Check sheet for the modelled part. Datum: model origin and axes. Units: mm. A direction names the side the tool comes from. Round coordinates to 2 decimals unless told otherwise and drop trailing zeros. Order: outer loops, then holes, each group sorted by start corner. A loop starts at its lowest first (then second) coordinate and runs counter-clockwise, first axis right, second up.
(1) Depth check by flat-ended pin: pin 1 (5 mm diameter, centred on x = -10.5, z = 37.5, fed in from -Y); pin 2 (12 mm diameter, centred on x = -43.5, z = 7.5, fed in from +Y). Enter the tip coordinate at first touch or a pass-through.
(2) Thickness scan on probe 1 along Z at (x, y) = (-9, 74); probe 2 along Z at (x, y) = (-75, 3); probe 3 along Y at (x, z) = (-89.5, 12.5). Record the ranges inside material, lowest first.
(3) Sectioned sample at D-D, the plane z = 8. Enter the section's corners in (x, y).
(4) Mould release check, pull along X, two halves, no side actions. Record for faces 1 (the flat face through (-17, 35, 60)), 2 (the flat face through (-15, 15, 30)), 3 (the flat face through (0, 44, 9)): released by +X, released by -X, zero draft, split by the parting line, or undercut.
(5) Sectioned sample at A-A, the plane x = -75. Enter the section's corners in (y, z).
(6) Tool access check on faces 4 (the flat face through (-20, 51, 30)), 5 (the flat face through (-12, 90, 30)), 6 (the cylindrical face through (-17.496, 20.07, 30.385)). Record the directions out of +Z, -Z, +X, -X, +Y, -Y that give a thin tool (end or side, any length) a straight path to the whole face; none if there is none.
(7) Sectioned sample at B-B, the plane z = 40. Enter the section's corners in (x, y), and give its area (3 significant figures).
(8) Sectioned sample at C-C, the plane y = 37. Enter the section's corners in (x, z), and give its area (3 significant figures).
```python
from build123d import *

# Parameters (mm, degrees)
F1_DEPTH = 60
F3_DEPTH = 90.001
F4_R     = 3.75
F5_DEPTH = 10.001
F6_W     = 10
F6_H     = 3


with BuildPart() as f1:
    # F0 (on Top) → F1 (new body)
    with BuildSketch(Plane.XY):
        Polygon((-100, 0), (0, 0), (0, 90), (-20, 90), (-20, 10), (-100, 10), align=None)
    extrude(amount=F1_DEPTH)

    # F2 (on face) → F3 (cut, through all)
    with BuildSketch(Plane(origin=(0, 90, 0), x_dir=(-1, 0, 0), z_dir=(0, 1, 0))):
        with BuildLine():
            ThreePointArc((0, 18.5), (8.131728, 21.868272), (11.5, 30))
            ThreePointArc((11.5, 30), (8.131728, 38.131728), (0, 41.5))
            Line((0, 41.5), (0, 18.5))
        make_face()
    extrude(amount=-F3_DEPTH, mode=Mode.SUBTRACT)

    # F4 (on face) → F5 (cut, through all)
    with BuildSketch(Plane(origin=(0, 10, 0), x_dir=(-1, 0, 0), z_dir=(0, 1, 0))):
        with Locations((75, 30)):
            Circle(F4_R)
    extrude(amount=-F5_DEPTH, mode=Mode.SUBTRACT)

    # F6 (on face) → F7 (revolve, cut)
    with BuildSketch(Plane.YZ):
        with Locations((70, 46)):
            Rectangle(F6_W, F6_H)
        with Locations((20, 46)):
            Rectangle(F6_W, F6_H)
    revolve(axis=Axis((0, 45, 30), (0, -1, 0)), mode=Mode.SUBTRACT)


solid = f1.part
```
Derived:
1. pin 1: stops at y = 0
1. pin 2: stops at y = 10
2. probe 1: z = 0 to 14.99, 18.63 to 22.84, 37.16 to 41.37, 45.01 to 60
2. probe 2: z = 0 to 26.25, 33.75 to 60
2. probe 3: y = 0 to 10
3. outline: (-100, 0) - (0, 0) - (0, 90) - (-20, 90) - (-20, 10) - (-100, 10) - close
4. face 1: zero draft
4. face 2: undercut
4. face 3: released by +X
5. outline: (0, 0) - (10, 0) - (10, 26.25) - (0, 26.25) - close; (0, 33.75) - (10, 33.75) - (10, 60) - (0, 60) - close
6. face 4: +Z, -Z, -X, +Y
6. face 5: +Z, -Z, +X, -X, +Y
6. face 6: none
7. outline: (-100, 0) - (-5.68, 0) - (-5.68, 90) - (-20, 90) - (-20, 10) - (-100, 10) - close; hole (-14.36, 15) - (-10.5, 15) - (-10.5, 25) - (-14.36, 25) - close; hole (-14.36, 65) - (-10.5, 65) - (-10.5, 75) - (-14.36, 75) - close
7. area: 2,010 mm2
8. outline: (-20, 0) - (0, 0) - (0, 18.5) arc R11.5 cw to (0, 41.5) - (0, 60) - (-20, 60) - close
8. area: 992 mm2
